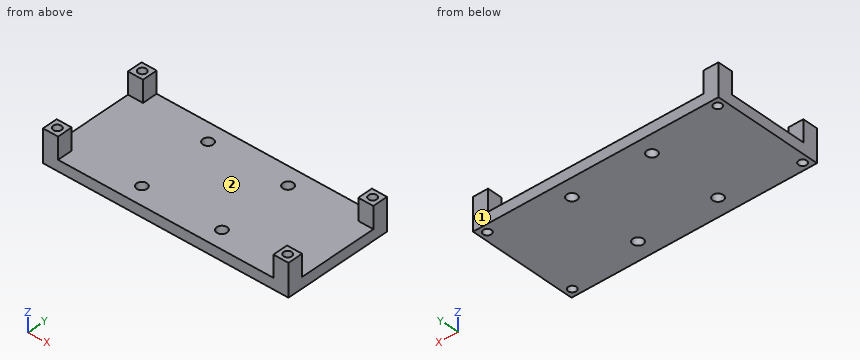
from build123d import *

# Parameters (mm, degrees)
SKETCH2_R           = 0.95
SKETCH2_R_2         = 0.75
BOSS_EXTRUDE1_DEPTH = 2
SKETCH4_W           = 2.78
SKETCH4_H           = 2.78
SKETCH4_R           = 0.75
BOSS_EXTRUDE2_DEPTH = 4


with BuildPart() as part:
    # Sketch2 → Boss-Extrude1 (new body)
    with BuildSketch(Plane.XY):
        Polygon((36.99, 25.1), (-8.29, 25.1), (-8.29, 5), (3.35, 5), (25.35, 5), (36.99, 5), align=None)
        with Locations((6.967324962, 8.304919624)):
            Circle(SKETCH2_R, mode=Mode.SUBTRACT)
        with Locations(Location((6.967324962, 21.795080376, 0), (0, 0, 180))):
            Circle(SKETCH2_R, mode=Mode.SUBTRACT)
        with Locations(Location((21.732675038, 8.304919624, 0), (0, 0, 180))):
            Circle(SKETCH2_R, mode=Mode.SUBTRACT)
        with Locations((21.732675038, 21.795080376)):
            Circle(SKETCH2_R, mode=Mode.SUBTRACT)
        with Locations((35.6, 23.71)):
            Circle(SKETCH2_R_2, mode=Mode.SUBTRACT)
        with Locations((35.6, 6.39)):
            Circle(SKETCH2_R_2, mode=Mode.SUBTRACT)
        with Locations((-6.9, 6.39)):
            Circle(SKETCH2_R_2, mode=Mode.SUBTRACT)
        with Locations((-6.9, 23.71)):
            Circle(SKETCH2_R_2, mode=Mode.SUBTRACT)
    extrude(amount=BOSS_EXTRUDE1_DEPTH)

    # Sketch4 → Boss-Extrude2 (add)
    # profile 1 of 4: a face of its own
    with BuildSketch(Plane.XY.offset(2)):
        with Locations((-6.9, 23.71)):
            Rectangle(SKETCH4_W, SKETCH4_H)
        with Locations((-6.9, 23.71)):
            Circle(SKETCH4_R, mode=Mode.SUBTRACT)
    # profile 2 of 4: a face of its own
    with BuildSketch(Plane.XY.offset(2)):
        with Locations((35.6, 23.71)):
            Rectangle(SKETCH4_W, SKETCH4_H)
        with Locations(Location((35.6, 23.71, 0), (0, 0, 180))):
            Circle(SKETCH4_R, mode=Mode.SUBTRACT)
    # profile 3 of 4: a face of its own
    with BuildSketch(Plane.XY.offset(2)):
        with Locations((35.6, 6.39)):
            Rectangle(SKETCH4_W, SKETCH4_H)
        with Locations((35.6, 6.39)):
            Circle(SKETCH4_R, mode=Mode.SUBTRACT)
    # profile 4 of 4: a face of its own
    with BuildSketch(Plane.XY.offset(2)):
        with Locations((-6.9, 6.39)):
            Rectangle(SKETCH4_W, SKETCH4_H)
        with Locations(Location((-6.9, 6.39, 0), (0, 0, 180))):
            Circle(SKETCH4_R, mode=Mode.SUBTRACT)
    extrude(amount=BOSS_EXTRUDE2_DEPTH)


solid = part.part
Verification items for the finished model (mm, model axes). Face numbers are marked on the shaded views. Coordinates: 2 decimals unless noted, no trailing zeros. Loops run counter-clockwise (first coordinate to the right, second up) from the corner with the lowest first, then second, coordinate; pieces in that order, holes last. Notation, with made-up numbers: M 18.5,78 L 57.5,78 A18 cw 57.5,104 Z; hole C 87,12.25 d1. An arc over 180 degrees is marked long. One line per item, written item: value.
1. Gauge pin test, flat ends, axial feed: P1, Ø0.9, axis at x = 35.6, y = 6.39, coming from the -Z side; P2, Ø10, axis at x = 18, y = 17, coming from the +Z side. Record the tip position at first contact, or that the pin passes through.
Answers follow:
P1: through
P2: z = 2
2. Section check B-B on x = -6.9. Record the cut outline in (y, z).
Answers follow:
outline: M 5,0 L 5.64,0 L 5.64,6 L 5,6 Z; M 7.14,0 L 22.96,0 L 22.96,6 L 22.32,6 L 22.32,2 L 7.78,2 L 7.78,6 L 7.14,6 Z; M 24.46,0 L 25.1,0 L 25.1,6 L 24.46,6 Z
3. Section check D-D on z = 0.4. Give the number of separate pieces and of enclosed holes in the cut face, plus the area to 3 significant figures.
Answers follow:
separate pieces: 1
enclosed holes: 8
area: 892 mm^2
4. Mould release check, pull along X, two halves, no side actions. Record for the marked faces 1 and 2: pulls with the +X half, pulls with the -X half, needs draft (parallel to the pull), parting line crosses it, or undercut.
Answers follow:
face 1: needs draft
face 2: undercut
5. Section check C-C on y = 6.39. Record the cut outline in (x, z), plus the area to 3 significant figures.
Answers follow:
outline: M -8.29,0 L -7.65,0 L -7.65,6 L -8.29,6 Z; M -6.15,0 L 34.85,0 L 34.85,6 L 34.21,6 L 34.21,2 L -5.51,2 L -5.51,6 L -6.15,6 Z; M 36.35,0 L 36.99,0 L 36.99,6 L 36.35,6 Z
area: 94.8 mm^2
6. Material ranges on line 1 along X through (y, z) = (23.75, 2.05); line 2 along Y through (x, z) = (-6.9, 1.45); line 3 along Z through (x, y) = (7, 17.5), recorded low to high. Write a range as from..to.
Answers follow:
line 1: -8.29..-7.65, -6.15..-5.51, 34.21..34.85, 36.35..36.99
line 2: 5..5.64, 7.14..22.96, 24.46..25.1
line 3: 0..2
7. Section check A-A on z = 3.5. Record the cut outline in (x, y), plus the area to 3 significant figures.
Answers follow:
outline: M -8.29,5 L -5.51,5 L -5.51,7.78 L -8.29,7.78 Z; M -8.29,22.32 L -5.51,22.32 L -5.51,25.1 L -8.29,25.1 Z; M 34.21,5 L 36.99,5 L 36.99,7.78 L 34.21,7.78 Z; M 34.21,22.32 L 36.99,22.32 L 36.99,25.1 L 34.21,25.1 Z; hole C -6.9,6.39 d1.5; hole C -6.9,23.71 d1.5; hole C 35.6,6.39 d1.5; hole C 35.6,23.71 d1.5
area: 23.8 mm^2
